Source: CAD feature listing. Evaluate the final solid. Frame: model axes, mm. Round coordinates to 2 decimals unless told otherwise and drop trailing zeros. Loops run counter-clockwise (first coordinate to the right, second up) from the corner with the lowest first, then second, coordinate; pieces in that order, holes last. Notation, with made-up numbers: M -24,65.25 L 28,65.25 A21 ccw 28,72.25 Z; hole C -18.75,56.5 d3. An arc over 180 degrees is marked long. Write each question's results on one line, items separated by ' | '. Start each with the question number.
1. Section C-C on y = -2. Give the number of separate pieces and of enclosed holes in the cut face, and give its area (3 significant figures).
2. Contact query for a flat-ended pin moving along its axis: pin 1 Ø5 at (x, z) = (19.35, 19.35) entering from +Y (3 decimals). Output: stop coordinate, or through.
3. Ray query, line 1 (X direction, y = 3, z = 166); line 2 (Z direction, x = -14, y = -0.5); line 3 (Z direction, x = -16, y = 1). Return the intervals inside material, ascending.
4. Section D-D on z = 72.5. Output: boundary loops of the cut face in (x, y) (3 decimals).
5. Section A-A on x = 0. Output: boundary loops of the cut face in (y, z) (3 decimals).
6. Section B-B on z = 173.5. Output: boundary loops of the cut face in (x, y) (3 decimals), and give its area (3 significant figures).
from build123d import *

# Parameters (mm, degrees)
BOSS_EXTRUDE1_DEPTH = 3.175
SKETCH2_R           = 21.5
CUT_EXTRUDE1_DEPTH  = 215.322525648
SKETCH3_W           = 42
SKETCH3_H           = 55.35
CUT_EXTRUDE2_DEPTH  = 215.322525648
SKETCH4_R           = 1.5
CUT_EXTRUDE3_DEPTH  = 215.322525648
FILLET1_R           = 10
SKETCH5_R           = 2
CUT_EXTRUDE4_DEPTH  = 215.322525648
CUT_EXTRUDE5_DEPTH  = 215.322525648
FILLET2_R           = 76
SKETCH7_R           = 1.55
CUT_EXTRUDE6_DEPTH  = 10


with BuildPart() as part:
    # Sketch1 → Boss-Extrude1 (new, symmetric)
    with BuildSketch(Plane(origin=(0, 0, 0), x_dir=(1, 0, 0), z_dir=(0, 1, 0))):
        with BuildLine():
            Line((35, -211.35), (35, 0))
            ThreePointArc((35, 0), (0, 35), (-35, 0))
            Line((-35, 0), (-35, -211.35))
            Line((-35, -211.35), (35, -211.35))
        make_face()
    extrude(amount=BOSS_EXTRUDE1_DEPTH, both=True)

    # Sketch2 → Cut-Extrude1 (cut, through all)
    with BuildSketch(Plane(origin=(0, 3.175, 0), x_dir=(1, 0, 0), z_dir=(0, 1, 0))):
        with Locations(Location((0, 0, 0), (0, 0, 270))):
            Circle(SKETCH2_R)
    extrude(amount=-CUT_EXTRUDE1_DEPTH, mode=Mode.SUBTRACT)

    # Sketch3 → Cut-Extrude2 (cut, through all)
    with BuildSketch(Plane(origin=(0, 3.175, 0), x_dir=(1, 0, 0), z_dir=(0, 1, 0))):
        with Locations((0, -162.325)):
            Rectangle(SKETCH3_W, SKETCH3_H)
    extrude(amount=-CUT_EXTRUDE2_DEPTH, mode=Mode.SUBTRACT)

    # Sketch4 → Cut-Extrude3 (cut, through all)
    with BuildSketch(Plane.XZ.offset(3.175)):
        with Locations(Location((-19.35, 19.35, 0), (0, 0, 270))):
            Circle(SKETCH4_R)
        with Locations(Location((19.35, 19.35, 0), (0, 0, 270))):
            Circle(SKETCH4_R)
        with Locations(Location((19.35, -19.35, 0), (0, 0, 270))):
            Circle(SKETCH4_R)
        with Locations(Location((-19.35, -19.35, 0), (0, 0, 270))):
            Circle(SKETCH4_R)
    extrude(amount=-CUT_EXTRUDE3_DEPTH, mode=Mode.SUBTRACT)

    # Fillet1
    fillet1_edges = [part.edges().sort_by_distance(p)[0] for p in [
        (35, 0, 211.35),
        (-35, 0, 211.35),
    ]]
    fillet(fillet1_edges, radius=FILLET1_R)

    # Sketch5 → Cut-Extrude4 (cut, through all)
    with BuildSketch(Plane(origin=(0, 3.175, 0), x_dir=(1, 0, 0), z_dir=(0, 1, 0))):
        with Locations(Location((15, -65.35, 0), (0, 0, 270))):
            Circle(SKETCH5_R)
        with Locations(Location((-15, -65.35, 0), (0, 0, 270))):
            Circle(SKETCH5_R)
        with Locations(Location((27.5, -195.35, 0), (0, 0, 270))):
            Circle(SKETCH5_R)
        with Locations(Location((-27.5, -195.35, 0), (0, 0, 270))):
            Circle(SKETCH5_R)
    extrude(amount=-CUT_EXTRUDE4_DEPTH, mode=Mode.SUBTRACT)

    # Sketch6 → Cut-Extrude5 (cut, through all)
    with BuildSketch(Plane(origin=(0, 3.175, 0), x_dir=(1, 0, 0), z_dir=(0, 1, 0))):
        with BuildLine():
            Line((-35, -134.65), (-35, -49.65))
            ThreePointArc((-35, -49.65), (-18.102907984, -92.15), (-35, -134.65))
        make_face()
    cut_extrude5 = extrude(amount=-CUT_EXTRUDE5_DEPTH, mode=Mode.SUBTRACT)

    # Mirror1: Cut-Extrude5 across plane
    add(cut_extrude5.mirror(Plane(origin=(0, 0, 0), x_dir=(0, 0, 1), z_dir=(1, 0, 0))), mode=Mode.SUBTRACT)

    # Fillet2
    fillet2_edges = [part.edges().sort_by_distance(p)[0] for p in [
        (35, 0, 134.65),
        (35, 0, 49.65),
        (-35, 0, 49.65),
        (-35, 0, 134.65),
    ]]
    fillet(fillet2_edges, radius=FILLET2_R)

    # Sketch7 → Cut-Extrude6 (cut)
    with BuildSketch(Plane(origin=(0, 3.175, 0), x_dir=(1, 0, 0), z_dir=(0, 1, 0))):
        with Locations(Location((-19.25, -205.675, 0), (0, 0, 270))):
            Circle(SKETCH7_R)
        with Locations(Location((19.25, -205.675, 0), (0, 0, 270))):
            Circle(SKETCH7_R)
    extrude(amount=-CUT_EXTRUDE6_DEPTH, mode=Mode.SUBTRACT)


solid = part.part
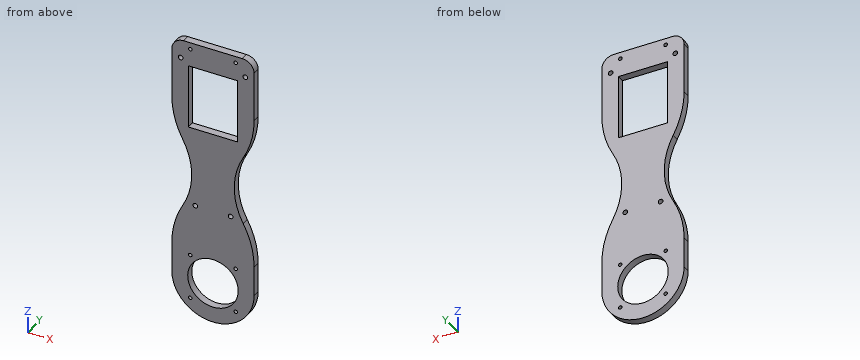
Taken from the geometry:
1) separate pieces: 1 | enclosed holes: 12 | area: 10,700 mm^2
2) pin 1: y = 3.175
3) line 1: -35 to -21, 21 to 35 | line 2: -32.08 to -16.32, 16.32 to 63.62, 67.08 to 134.65, 190 to 211.35 | line 3: -31.13 to -14.36, 14.36 to 63.62, 67.08 to 134.65, 190 to 211.35
4) outline: M -21.305,-3.175 L 21.305,-3.175 L 21.305,3.175 L -21.305,3.175 Z
5) outline: M -3.175,-35 L 3.175,-35 L 3.175,-21.5 L -3.175,-21.5 Z; M -3.175,21.5 L 3.175,21.5 L 3.175,134.65 L -3.175,134.65 Z; M -3.175,190 L 3.175,190 L 3.175,211.35 L -3.175,211.35 Z
6) outline: M -35,-3.175 L -21,-3.175 L -21,3.175 L -35,3.175 Z; M 21,-3.175 L 35,-3.175 L 35,3.175 L 21,3.175 Z | area: 178 mm^2
